The figure shows three views and two pictorial views of one solid part (mm, origin at its lowest corner). Answer the questions. Give positions to 0.01 mm unless a question says otherwise; leave off trailing zeros. Loops run counter-clockwise (first coordinate to the right, second up) from the corner with the lowest first, then second, coordinate; pieces in that order, holes last. Notation, with made-up numbers: M 33.5,45 L 43.5,45 A28 cw 43.5,76 Z; hole C 5.5,-1 d8. An arc over 180 degrees is marked long. Write item = value, one per line. Start each with the question number.
1. A flat-ended cylindrical pin translates along its axis: pin 1 Ø4 at (y, z) = (8.5, 160) entering from -X (3 decimals). Find the tip coordinate at first contact, or state that the pin passes through.
2. Section B-B on z = 95 is taken. Determine the outline of the cut face in (x, y) (3 decimals).
3. Section C-C on y = 8.5 is taken. Determine the outline of the cut face in (x, z) (3 decimals).
4. Consider L1, parallel to Y at x = 15.5, z = 120.5 (3 decimals); L2, parallel to X at y = 5.75, z = 179 (3 decimals). Determine where each line is inside the solid, lowest interval first. Write a range as [from, to].
5. Section A-A on x = 11.25 is taken. Determine the outline of the cut face in (y, z) (3 decimals).
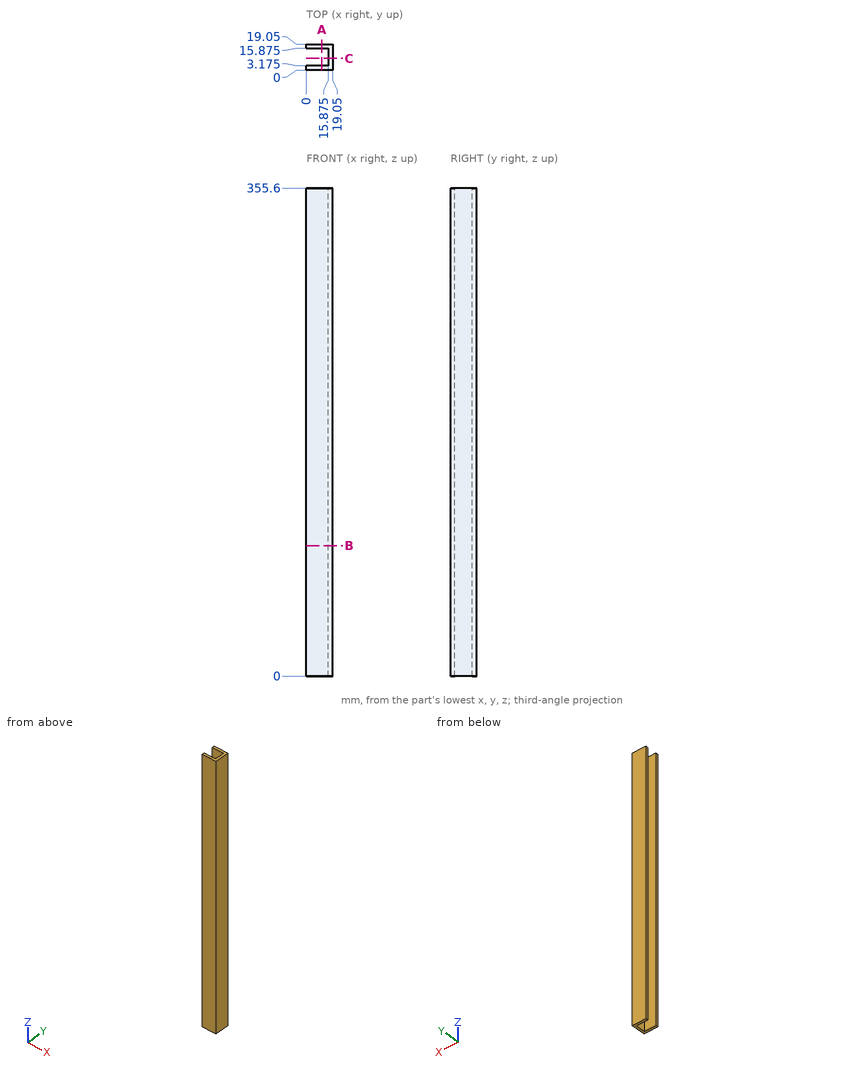
Verdict:
q1.pin_1 = 15.875
q2.outline = M 0,0 L 19.05,0 L 19.05,19.05 L 0,19.05 L 0,15.875 L 15.875,15.875 L 15.875,3.175 L 0,3.175 Z
q3.outline = M 15.875,0 L 19.05,0 L 19.05,355.6 L 15.875,355.6 Z
q4.L1 = [0, 3.175], [15.875, 19.05]
q4.L2 = [15.875, 19.05]
q5.outline = M 0,0 L 3.175,0 L 3.175,355.6 L 0,355.6 Z; M 15.875,0 L 19.05,0 L 19.05,355.6 L 15.875,355.6 Z
